```python
from build123d import *

# Parameters (mm, degrees)
F1_DEPTH = 3.175
F3_D     = 3.175
F5_D     = 8


with BuildPart() as f1:
    # F0 (on Top) → F1 (new body)
    with BuildSketch(Plane.XY):
        Polygon((0, 25.4), (0, 0), (25.4, 0), (25.4, -101.6), (50.8, -101.6), (50.8, 0), (76.2, 0), (76.2, 25.4), align=None)
    extrude(amount=F1_DEPTH)

    # F3 (through all)
    with Locations(Plane.XY.offset(3.175)):
        with Locations((12.7, 12.7), (25.4, 12.7), (50.8, 12.7), (63.5, 12.7), (38.1, -25.4), (38.1, -50.8), (38.1, -76.2)):
            Hole(F3_D / 2)

    # F5 (through all)
    with Locations(Plane.XY.offset(3.175)):
        with Locations((38.1, 12.7)):
            Hole(F5_D / 2)


solid = f1.part
```
The listing builds one solid part. Answer for the finished solid, in the listing's coordinates (mm). A direction names the side the tool comes from. Coordinates: 2 decimals unless noted, no trailing zeros. Loops run counter-clockwise (first coordinate to the right, second up) from the corner with the lowest first, then second, coordinate; pieces in that order, holes last. Notation, with made-up numbers: M 38,4 L 80,4 A35 ccw 80,41 Z; hole C -28,37 d5. An arc over 180 degrees is marked long. Answer as a JSON object with one key per item and string values. Group by question number.
Item 1: Which of the six approach directions +Z, -Z, +X, -X, +Y, -Y give full straight-line access (tool end or side, diameter ignored) to faces 1 (the face through (37.37, -52.21, 1.57)), 2 (the face through (63, 0, 2)), 3 (the face through (13, 0, 2))?
Item 2: Section D-D (x = 69.5) is taken. Write down the section's boundary in (y, z) (3 decimals), and give its area (3 significant figures).
Item 3: Consider L1, parallel to Y at x = 38.1, z = 1; L2, parallel to Y at x = 63.5, z = 2.3; L3, parallel to X at y = -76.2, z = 2. Determine where each line is inside the solid, lowest interval first.
Item 4: Section B-B (x = 12.7) is taken. Write down the section's boundary in (y, z) (1 decimal), and give its area (3 significant figures).
Item 5: Determine the mould class of faces 4 (the face through (11.186, 13.177, 1.565)), 5 (the face through (39, 25.4, 2)), 6 (the face through (50.8, -52, 2)), 7 (the face through (26.57, 13.773, 1.565)) for opening direction X: +X half, -X half, draft (parallel to the pull), parting line (faces both ways), or undercut.
Item 6: Section A-A (y = -76.2) is taken. Write down the section's boundary in (x, z) (1 decimal).
Item 7: Section C-C (z = 2) is taken. Give the number of separate pieces and of enclosed holes in the cut face, and give its area (3 significant figures).
Item 8: Each of these flat-tipped pins is pushed along its axis until it touches: P1, Ø3, axis at x = 38.1, y = -50.8, coming from the +Z side; P2, Ø1.6, axis at y = -36, z = 2, coming from the -X side; P3, Ø1.5, axis at y = -47.5, z = 0.5, coming from the +X side. Where does it stop, or does it pass through?
Solved:
{
 "1": {"face 1": "+Z, -Z", "face 2": "+Z, -Z, +X, -Y", "face 3": "+Z, -Z, -X, -Y"},
 "2": {"outline": "M 0,0 L 25.4,0 L 25.4,3.175 L 0,3.175 Z", "area": "80.6 mm2"},
 "3": {"L1": "y = -101.6 to -77.79, -74.61 to -52.39, -49.21 to -26.99, -23.81 to 8.7, 16.7 to 25.4", "L2": "y = 0 to 11.11, 14.29 to 25.4", "L3": "x = 25.4 to 36.51, 39.69 to 50.8"},
 "4": {"outline": "M 0,0 L 11.1,0 L 11.1,3.2 L 0,3.2 Z; M 14.3,0 L 25.4,0 L 25.4,3.2 L 14.3,3.2 Z", "area": "70.6 mm2"},
 "5": {"face 4": "undercut", "face 5": "draft", "face 6": "+X half", "face 7": "undercut"},
 "6": {"outline": "M 25.4,0 L 36.5,0 L 36.5,3.2 L 25.4,3.2 Z; M 39.7,0 L 50.8,0 L 50.8,3.2 L 39.7,3.2 Z"},
 "7": {"separate pieces": "1", "enclosed holes": "8", "area": "4,410 mm2"},
 "8": {"P1": "passes through", "P2": "stops at x = 25.4", "P3": "stops at x = 50.8"}
}
